Part model, mm, in its own coordinate system. A direction names the side the tool comes from. Round coordinates to 2 decimals unless told otherwise and drop trailing zeros. Write each loop counter-clockwise with the first axis right and the second up, starting at its lowest first coordinate (ties: lowest second). Pieces come first, ordered by that corner, then holes.
1) Which spindle directions (+Z, -Z, +X, -X, +Y, -Y) get a long thin tool onto all of the face, cutting with end or side? Do faces 1 (the flat face through (19, 279.4, 57)), 2 (the flat face through (19, 431.8, 57)), 3 (the flat face through (6.35, 355, 57)), 4 (the flat face through (19, -457.2, -1)), 5 (the flat face through (31.75, 355, 57)). Say none if no direction does.
2) Saw through at A-A on y = 325.5. Write the cut outline in (x, z).
3) Flat gauge pins, fed straight in: pin 1 (10 mm diameter, centred on x = 18.88, y = -317.5, fed in from +Z); pin 2 (1.5 mm diameter, centred on x = 15.5, z = 55.5, fed in from -Y); pin 3 (12.5 mm diameter, centred on y = 339, z = 53, fed in from -X). Where does each tip first touch, or does it go through?
4) Drill centre lines: L1, parallel to X at y = -317.5, z = 28.25; L2, parallel to X at y = 286.5, z = 62; L3, parallel to Z at x = 3, y = 204. Where is each one in solid material? Low to high.
5) Saw through at B-B on z = 61.5. Write the cut outline in (x, y), and give its area (3 significant figures).
```python
from build123d import *

# Parameters (mm, degrees)
F0_W     = 914.4
F0_H     = 88.9
F1_DEPTH = 38.1
F2_R     = 6.35
F3_DEPTH = 25.4
F4_W     = 25.4
F4_H     = 152.4
F5_DEPTH = 25.4


with BuildPart() as f1:
    # F0 (on Right) → F1 (new body)
    with BuildSketch(Plane.YZ):
        Rectangle(F0_W, F0_H)
    extrude(amount=F1_DEPTH)

    # F2 (on face) → F3 (cut)
    with BuildSketch(Plane.XY.offset(44.45)):
        with Locations((18.882329, -317.5)):
            Circle(F2_R)
    extrude(amount=-F3_DEPTH, mode=Mode.SUBTRACT)

    # F4 (on face) → F5 (join)
    with BuildSketch(Plane.XY.offset(44.45)):
        with Locations((19.05, 355.6)):
            Rectangle(F4_W, F4_H)
    extrude(amount=F5_DEPTH)


solid = f1.part
```
Completed:
1. face 1: +Z, +X, -X, -Y
1. face 2: +Z, +X, -X, +Y
1. face 3: +Z, -X, +Y, -Y
1. face 4: +Z, -Z, +X, -X, -Y
1. face 5: +Z, +X, +Y, -Y
2. outline: (0, -44.45) - (38.1, -44.45) - (38.1, 44.45) - (31.75, 44.45) - (31.75, 69.85) - (6.35, 69.85) - (6.35, 44.45) - (0, 44.45) - close
3. pin 1: stops at z = 19.05
3. pin 2: stops at y = 279.4
3. pin 3: stops at x = 6.35
4. L1: x = 0 to 12.53, 25.23 to 38.1
4. L2: x = 6.35 to 31.75
4. L3: z = -44.45 to 44.45
5. outline: (6.35, 279.4) - (31.75, 279.4) - (31.75, 431.8) - (6.35, 431.8) - close
5. area: 3,870 mm2
